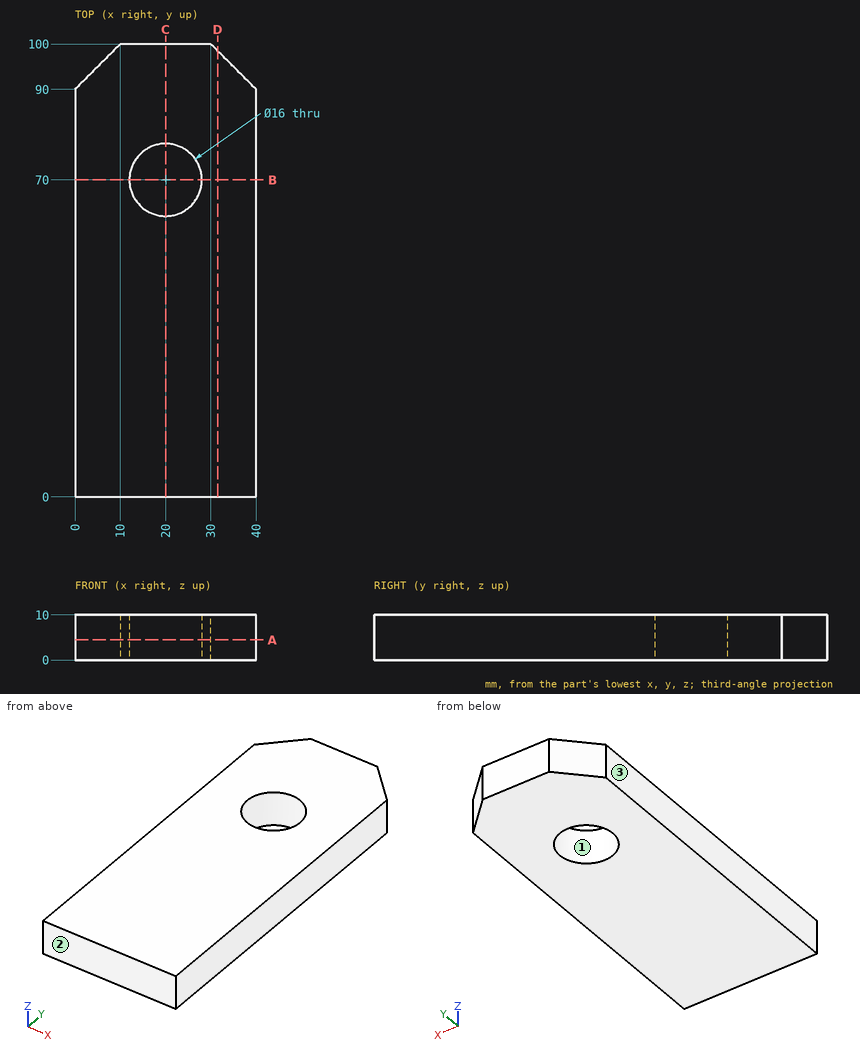
Geometry: see drawing. Coordinates: mm, zero at the bounding-box minimum. Give positions to 0.01 mm unless a question says otherwise; leave off trailing zeros. Order: outer loops, then holes, each group sorted by start corner. A loop starts at its lowest first (then second) coordinate and runs counter-clockwise, first axis right, second up. Notation, with made-up numbers: (-38.75, 64) -> (-20.75, 64) arc R8 ccw to (-20.75, 75) -> close; hole circle Ø3 at (-17.5, -37.5). An arc over 180 degrees is marked (long way). Write item = value, one per line.
Q1. Cut plane C-C, the plane x = 20. Output: boundary loops of the cut face in (y, z), and give its area (3 significant figures).
Data:
outline = (0, 0) -> (62, 0) -> (62, 10) -> (0, 10) -> close; (78, 0) -> (100, 0) -> (100, 10) -> (78, 10) -> close
area = 840 mm^2
Q2. Material intervals for line 1 (Y direction, x = 20, z = 4); line 2 (Y direction, x = 21, z = 8.5); line 3 (X direction, y = 68, z = 3), sorted ascending. Write a range as from..to.
Data:
line_1 = 0..62, 78..100
line_2 = 0..62.06, 77.94..100
line_3 = 0..12.25, 27.75..40
Q3. Cut plane B-B, the plane y = 70. Output: boundary loops of the cut face in (x, z).
Data:
outline = (0, 0) -> (12, 0) -> (12, 10) -> (0, 10) -> close; (28, 0) -> (40, 0) -> (40, 10) -> (28, 10) -> close
Q4. Pull-direction query (Y, two-part tool) for the marked faces 1, 2 and 3; classes: released by +Y, released by -Y, zero draft, split by the parting line, or undercut.
Data:
face_1 = undercut
face_2 = released by -Y
face_3 = zero draft
Q5. Cut plane A-A, the plane z = 4.5. Output: boundary loops of the cut face in (x, y), and give its area (3 significant figures).
Data:
outline = (0, 0) -> (40, 0) -> (40, 90) -> (30, 100) -> (10, 100) -> (0, 90) -> close; hole circle Ø16 at (20, 70)
area = 3,700 mm^2
Q6. Cut plane D-D, the plane x = 31.5. Output: boundary loops of the cut face in (y, z).
Data:
outline = (0, 0) -> (98.5, 0) -> (98.5, 10) -> (0, 10) -> close
Q7. Pin query (flat end, axial travel): pin 1 (3 mm diameter, centred on y = 34.5, z = 6, fed in from -X). Return the tip coordinate at first contact, or that it passes through.
Data:
pin_1 = 0
